```python
from build123d import *

# Parameters (mm, degrees)
BOSS_EXTRUDE1_DEPTH = 5
SKETCH3_W           = 21.5
SKETCH3_H           = 20
SKETCH3_R           = 1
BOSS_EXTRUDE2_DEPTH = 5


with BuildPart() as part:
    # Sketch1 → Boss-Extrude1 (new body)
    with BuildSketch(Plane(origin=(0, 0, 0), x_dir=(1, 0, 0), z_dir=(0, 1, 0))):
        with BuildLine():
            Line((25, 25), (201.409203428, 25))
            Line((201.409203428, 25), (201.409203428, 40))
            Line((201.409203428, 40), (207.876498783, 40))
            add(Edge.make_bspline(
                [(207.876498783, -40), (239.223771283, 0), (207.876498783, 40)],
                knots=[2.771189847, 2.771189847, 2.771189847, 3.51199546, 3.51199546, 3.51199546], degree=2, weights=[1, 0.932181609, 1]))
            Line((207.876498783, -40), (201.409203428, -40))
            Line((201.409203428, -40), (201.409203428, -25))
            Line((201.409203428, -25), (25, -25))
            Line((25, -25), (25, -109.803415805))
            add(Edge.make_bspline(
                [(-25, -109.803415805), (0, -111.20100327), (25, -109.803415805)],
                knots=[1.458452535, 1.458452535, 1.458452535, 1.683140119, 1.683140119, 1.683140119], degree=2, weights=[1, 0.993696071, 1]))
            Line((-25, -109.803415805), (-25, -25))
            Line((-25, -25), (-201.409203425, -25))
            Line((-201.409203425, -25), (-201.409203425, -40))
            Line((-201.409203425, -40), (-207.876498783, -40))
            add(Edge.make_bspline(
                [(-207.876498783, 40), (-239.223771283, 0), (-207.876498783, -40)],
                knots=[5.912782501, 5.912782501, 5.912782501, 6.653588114, 6.653588114, 6.653588114], degree=2, weights=[1, 0.932181609, 1]))
            Line((-207.876498783, 40), (-201.409203425, 40))
            Line((-201.409203425, 40), (-201.409203425, 25))
            Line((-201.409203425, 25), (-25, 25))
            Line((-25, 25), (-25, 109.803415805))
            add(Edge.make_bspline(
                [(25, 109.803415805), (0, 111.20100327), (-25, 109.803415805)],
                knots=[4.600045189, 4.600045189, 4.600045189, 4.824732772, 4.824732772, 4.824732772], degree=2, weights=[1, 0.993696071, 1]))
            Line((25, 109.803415805), (25, 25))
        make_face()
    extrude(amount=BOSS_EXTRUDE1_DEPTH)

    # Sketch3 → Boss-Extrude2 (add)
    # profile 1 of 2: a face of its own
    with BuildSketch(Plane(origin=(0, 5, 0), x_dir=(1, 0, 0), z_dir=(0, 1, 0))):
        Polygon((-25, -60), (-36.5, -60), (-46.5, -60), (-46.5, -80), (-25, -80), align=None)
        with BuildLine():
            ThreePointArc((-35.5, -70), (-37.207106781, -70.707106781), (-36.5, -69))
            ThreePointArc((-36.5, -69), (-35.792893219, -69.292893219), (-35.5, -70))
        make_face(mode=Mode.SUBTRACT)
    # profile 2 of 2: a face of its own
    with BuildSketch(Plane(origin=(0, 5, 0), x_dir=(1, 0, 0), z_dir=(0, 1, 0))):
        with Locations((35.75, -70)):
            Rectangle(SKETCH3_W, SKETCH3_H)
        with Locations(Location((36.5, -70, 0), (0, 0, 270))):
            Circle(SKETCH3_R, mode=Mode.SUBTRACT)
    extrude(amount=-BOSS_EXTRUDE2_DEPTH)


solid = part.part
```
Verification items for the finished model (mm, model axes). Give positions to 0.01 mm unless a question says otherwise; leave off trailing zeros. Loops run counter-clockwise (first coordinate to the right, second up) from the corner with the lowest first, then second, coordinate; pieces in that order, holes last. Notation, with made-up numbers: M 1,16.5 L 20,16.5 A27 ccw 20,50.5 Z; hole C 1.5,67.5 d6. An arc over 180 degrees is marked long. Return JSON: item names as keys, results as strings.
1) Section check A-A, the plane y = 1.65. Count the separate pieces of the cut face and the enclosed holes in it, and give its area (3 significant figures).
Findings:
{"separate pieces": "1", "enclosed holes": "2", "area": "32,200 mm2"}
2) Section check C-C, the plane z = -57. Enter the section's corners in (x, y), and give its area (3 significant figures).
Findings:
{"outline": "M -25,0 L 25,0 L 25,5 L -25,5 Z", "area": "250 mm2"}
3) Section check B-B, the plane x = 183. Enter the section's corners in (y, z).
Findings:
{"outline": "M 0,-25 L 5,-25 L 5,25 L 0,25 Z"}
4) Material ranges on L1, parallel to X at y = 2, z = 70; L2, parallel to Z at x = -36.5, y = 3.55; L3, parallel to X at y = 0.6, z = -31, recorded low to high. Write a range as [from, to].
Findings:
{"L1": "x = [-46.5, -37.5], [-35.5, 35.5], [37.5, 46.5]", "L2": "z = [-25, 25], [60, 69], [71, 80]", "L3": "x = [-214.04, -201.41], [-25, 25], [201.41, 214.04]"}
5) Gauge pin test, flat ends, axial feed: P1, Ø1, axis at y = 1.5, z = -3, coming from the -X side; P2, Ø3, axis at x = -36.5, z = 70, coming from the +Y side; P3, Ø2.5, axis at x = -121.5, y = 3, coming from the +Z side; P4, Ø1.5, axis at y = 3, z = 42, coming from the +X side. Record the tip position at first contact, or that the pin passes through.
Findings:
{"P1": "stops at x = -222.94", "P2": "stops at y = 5", "P3": "stops at z = 25", "P4": "stops at x = 25"}
